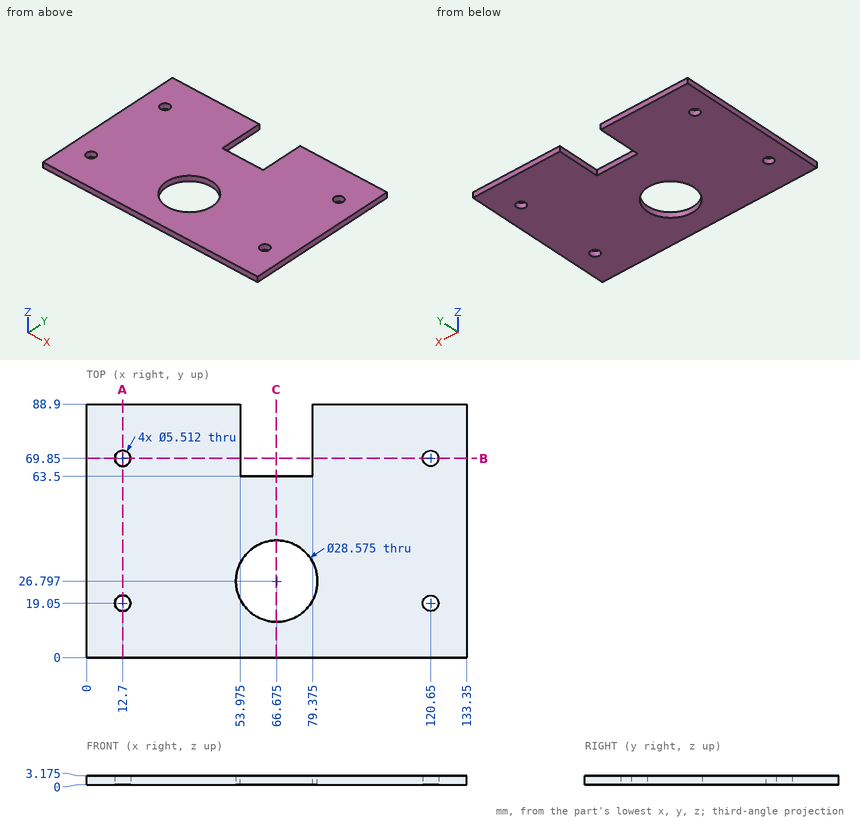
Study the drawing (mm; zero at the part's minimum x, y, z) and answer. Give positions to 0.01 mm unless a question says otherwise; leave off trailing zeros. Write each loop counter-clockwise with the first axis right and the second up, starting at its lowest first coordinate (ties: lowest second). Pieces come first, ordered by that corner, then holes. Notation, with made-up numbers: (-23.5, 3.5) - (32.5, 3.5) arc R24 cw to (32.5, 13.5) - close; hole circle Ø9 at (53.25, -3.5). An arc over 180 degrees is marked (long way). Write item = value, one per line. Start each with the question number.
Item 1: Find the intervals of material crossed by probe 1 along Y at (x, z) = (120.65, 1.2); probe 2 along X at (y, z) = (18, 2.5); probe 3 along X at (y, z) = (77, 0.8) (3 decimals), in increasing order. Write a range as [from, to].
Item 2: Find section A-A (x = 12.7). Give the vertices of the cut face in (y, z) (1 decimal).
Item 3: Find section B-B (y = 69.85). State how many separate pieces and enclosed holes the cut face has, then the cut area to 3 significant figures.
Item 4: Find section C-C (x = 66.5). Give the vertices of the cut face in (y, z) (1 decimal).
Item 5: Each of these flat-tipped pins is pushed along its axis until it touches: P1, Ø1.6, axis at x = 67, z = 2, coming from the +Y side; P2, Ø5, axis at x = 12.7, y = 69.85, coming from the +Z side. Where does it stop, or does it pass through?
Response:
q1.probe_1 = [0, 16.29], [21.81, 67.09], [72.61, 88.9]
q1.probe_2 = [0, 10.15], [15.25, 55.42], [77.93, 118.1], [123.2, 133.35]
q1.probe_3 = [0, 53.975], [79.375, 133.35]
q2.outline = (0, 0) - (16.3, 0) - (16.3, 3.2) - (0, 3.2) - close; (21.8, 0) - (67.1, 0) - (67.1, 3.2) - (21.8, 3.2) - close; (72.6, 0) - (88.9, 0) - (88.9, 3.2) - (72.6, 3.2) - close
q3.separate_pieces = 4
q3.enclosed_holes = 0
q3.area = 308 mm²
q4.outline = (0, 0) - (12.5, 0) - (12.5, 3.2) - (0, 3.2) - close; (41.1, 0) - (63.5, 0) - (63.5, 3.2) - (41.1, 3.2) - close
q5.P1 = 63.5
q5.P2 = through
